Work out the finished part from the listing and answer in its coordinate system (mm). Coordinates: 2 decimals unless noted, no trailing zeros. Write each loop counter-clockwise with the first axis right and the second up, starting at its lowest first coordinate (ties: lowest second). Pieces come first, ordered by that corner, then holes. Notation, with made-up numbers: (57, -34) - (85, -34) arc R23 cw to (85, -8) - close; hole circle Ø5 at (82, 43). An arc over 180 degrees is marked (long way). Use one line per item in the form item = value. Start each with the question number.
Item 1: Consider probe 1 along X at (y, z) = (0, 305); probe 2 along Y at (x, z) = (0, 297.6); probe 3 along Y at (x, z) = (0, 303). Determine where each line is inside the solid, lowest interval first.
Item 2: A cutting plane is placed at A-A (y = 63.5). Write down the section's boundary in (x, z), then the cut area to 3 significant figures.
Item 3: Given pin 1 (6.5 mm diameter, centred on x = 2.5, y = 1.5, fed in from -Z); pin 2 (0.6 mm diameter, centred on x = 7.5, y = 4.5, fed in from -Z), each flat-ended and moving along its own axis, determine where each tip first touches the part or whether it passes through.
Item 4: A cutting plane is placed at B-B (x = -45). Write down the section's boundary in (y, z).
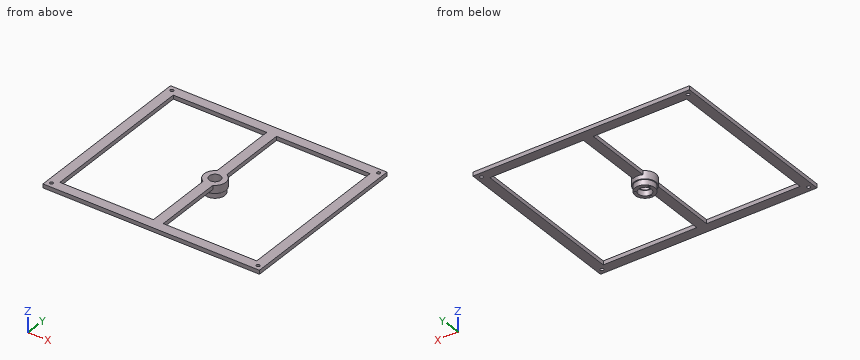
from build123d import *

# Parameters (mm, degrees)
UPPER_PERIMETER_START                         = 304
SKETCH1_W                                     = 220
SKETCH1_H                                     = 180
SKETCH1_W_2                                   = 200
SKETCH1_H_2                                   = 160
UPPER_PERIMETER_DEPTH                         = 4
BEARING_SPINE_START                           = 304
SKETCH2_W                                     = 10
SKETCH2_H                                     = 170
BEARING_SPINE_DEPTH                           = 4
UPPER_OUTER_RACE_STOP_START                   = 299.9
SKETCH3_R                                     = 11
SKETCH3_R_2                                   = 5.7
UPPER_OUTER_RACE_STOP_DEPTH                   = 8.1
FLOATING_OUTER_RACE_SEAT_START                = 294.5
SKETCH4_R                                     = 10
SKETCH4_R_2                                   = 6.5
FLOATING_OUTER_RACE_SEAT_DEPTH                = 5.41
SHAFT_CLIP_CLEARANCE_START                    = -8.11
SKETCH5_R                                     = 5.7
SHAFT_CLIP_CLEARANCE_DEPTH                    = 8.11
SKETCH6_R                                     = 1.7
FOUR_TIE_ROD_CLEARANCE_DEPTH                  = 4.01
SKETCH7_R                                     = 1
THREE_M2_TOP_CAP_THREAD_MAJOR_ENVELOPES_DEPTH = 4.3


with BuildPart() as part:
    # Sketch1 → Upper_Perimeter (new body)
    with BuildSketch(Plane.XY.offset(UPPER_PERIMETER_START)):
        Rectangle(SKETCH1_W, SKETCH1_H)
        Rectangle(SKETCH1_W_2, SKETCH1_H_2, mode=Mode.SUBTRACT)
    extrude(amount=UPPER_PERIMETER_DEPTH)

    # Sketch2 → Bearing_Spine (add)
    with BuildSketch(Plane.XY.offset(BEARING_SPINE_START)):
        Rectangle(SKETCH2_W, SKETCH2_H)
    extrude(amount=BEARING_SPINE_DEPTH)

    # Sketch3 → Upper_Outer_Race_Stop (add)
    with BuildSketch(Plane.XY.offset(UPPER_OUTER_RACE_STOP_START)):
        with Locations(Location((0, 0, 0), (0, 0, 117.035691789))):
            Circle(SKETCH3_R)
        with Locations(Location((0, 0, 0), (0, 0, 208.694413527))):
            Circle(SKETCH3_R_2, mode=Mode.SUBTRACT)
    extrude(amount=UPPER_OUTER_RACE_STOP_DEPTH)

    # Sketch4 → Floating_Outer_Race_Seat (add)
    with BuildSketch(Plane.XY.offset(FLOATING_OUTER_RACE_SEAT_START)):
        Circle(SKETCH4_R)
        Circle(SKETCH4_R_2, mode=Mode.SUBTRACT)
    extrude(amount=FLOATING_OUTER_RACE_SEAT_DEPTH)

    # Sketch5 → Shaft_Clip_Clearance (cut)
    with BuildSketch(Plane.XY.offset(308).offset(SHAFT_CLIP_CLEARANCE_START)):
        Circle(SKETCH5_R)
    extrude(amount=SHAFT_CLIP_CLEARANCE_DEPTH, mode=Mode.SUBTRACT)

    # Sketch6 → Four_Tie_Rod_Clearance (cut)
    with BuildSketch(Plane.XY.offset(308)):
        with Locations((-105, -85)):
            Circle(SKETCH6_R)
        with Locations((-105, 85)):
            Circle(SKETCH6_R)
        with Locations((105, -85)):
            Circle(SKETCH6_R)
        with Locations((105, 85)):
            Circle(SKETCH6_R)
    extrude(amount=-FOUR_TIE_ROD_CLEARANCE_DEPTH, mode=Mode.SUBTRACT)

    # Sketch7 → Three_M2_Top_Cap_Thread_Major_Envelopes (cut)
    with BuildSketch(Plane(origin=(0, 0, 294.5), x_dir=(-1, 0, 0), z_dir=(0, 0, -1))):
        with Locations((-7.188010851, 4.15)):
            Circle(SKETCH7_R)
        with Locations((7.188010851, 4.15)):
            Circle(SKETCH7_R)
        with Locations((0, -8.3)):
            Circle(SKETCH7_R)
    extrude(amount=-THREE_M2_TOP_CAP_THREAD_MAJOR_ENVELOPES_DEPTH, mode=Mode.SUBTRACT)


solid = part.part
Answer:
q1.probe_1 = -110 to -100, -11 to -5.7, 5.7 to 11, 100 to 110
q1.probe_2 = -10 to -9.3, -7.3 to -6.5, 6.5 to 10
q1.probe_3 = -11 to -5.7, 5.7 to 11
q2.outline = (-110, 304) - (-100, 304) - (-100, 308) - (-110, 308) - close; (-5, 304) - (5, 304) - (5, 308) - (-5, 308) - close; (100, 304) - (110, 304) - (110, 308) - (100, 308) - close
q2.area = 120 mm²
q3.pin_1 = 299.9
q3.pin_2 = 298.8
q4.outline = (-90, 304) - (-80, 304) - (-80, 308) - (-90, 308) - close; (80, 304) - (90, 304) - (90, 308) - (80, 308) - close
